from build123d import *

# Parameters (mm, degrees)
SKETCH1_W           = 180
SKETCH1_H           = 110
SKETCH1_R           = 42
SKETCH1_R_2         = 18.1
BOSS_EXTRUDE1_DEPTH = 6
SKETCH3_R           = 1
CUT_EXTRUDE1_DEPTH  = 30


with BuildPart() as part:
    # Sketch1 → Boss-Extrude1 (new body)
    with BuildSketch(Plane.XY):
        with Locations((90, 55)):
            Rectangle(SKETCH1_W, SKETCH1_H)
        with Locations((60, 50)):
            Circle(SKETCH1_R, mode=Mode.SUBTRACT)
        with Locations((140, 60)):
            Circle(SKETCH1_R_2, mode=Mode.SUBTRACT)
    extrude(amount=BOSS_EXTRUDE1_DEPTH)

    # Sketch3 → Cut-Extrude1 (cut)
    with BuildSketch(Plane.XY):
        with Locations((92.880465325, 82.880465325)):
            Circle(SKETCH3_R)
        with Locations((27.119534675, 82.880465325)):
            Circle(SKETCH3_R)
        with Locations((27.119534675, 17.119534675)):
            Circle(SKETCH3_R)
        with Locations((92.880465325, 17.119534675)):
            Circle(SKETCH3_R)
        with Locations((155.202795796, 75.202795796)):
            Circle(SKETCH3_R)
        with Locations((124.797204204, 75.202795796)):
            Circle(SKETCH3_R)
        with Locations((124.797204204, 44.797204204)):
            Circle(SKETCH3_R)
        with Locations((155.202795796, 44.797204204)):
            Circle(SKETCH3_R)
    extrude(amount=CUT_EXTRUDE1_DEPTH, mode=Mode.SUBTRACT)


solid = part.part
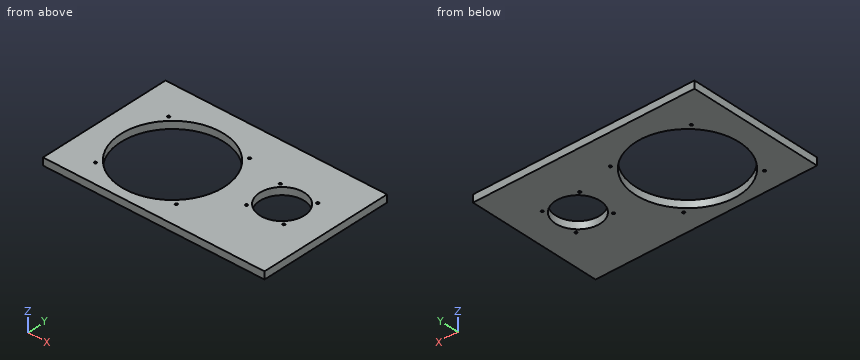
CAD build for the part. Positions are in the model's coordinates, mm. Give positions to 0.01 mm unless a question says otherwise; leave off trailing zeros. Loops run counter-clockwise (first coordinate to the right, second up) from the corner with the lowest first, then second, coordinate; pieces in that order, holes last. Notation, with made-up numbers: M 9,-31.75 L 66,-31.75 A26 cw 66,5.25 Z; hole C 64,48 d4. An arc over 180 degrees is marked long. Write each question's results on one line, items separated by ' | '.
Q1. Band-saw the part on B-B on y = 38. Write the cut outline in (x, z), and give its area (3 significant figures).
Geometry check:
outline: M 0,0 L 19.75,0 L 19.75,6 L 0,6 Z; M 100.25,0 L 180,0 L 180,6 L 100.25,6 Z | area: 597 mm²
Q2. Probe probe 1 along Y at (x, z) = (60, 2.85); probe 2 along Y at (x, z) = (155, 5.45); probe 3 along X at (y, z) = (68.5, 0.7). List the from-to ranges inside material, lowest first.
Geometry check:
probe 1: y = 0 to 8, 92 to 110 | probe 2: y = 0 to 43.82, 45.78 to 49.87, 70.13 to 74.22, 76.18 to 110 | probe 3: x = 0 to 22.29, 97.71 to 124.02, 155.98 to 180
Q3. Band-saw the part on C-C on z = 4.25. Give the number of separate pieces and of enclosed holes in the cut face, and give its area (3 significant figures).
Geometry check:
separate pieces: 1 | enclosed holes: 10 | area: 13,200 mm²
Q4. Band-saw the part on D-D on y = 50. Write the cut outline in (x, z), and give its area (3 significant figures).
Geometry check:
outline: M 0,0 L 18,0 L 18,6 L 0,6 Z; M 102,0 L 124.91,0 L 124.91,6 L 102,6 Z; M 155.09,0 L 180,0 L 180,6 L 155.09,6 Z | area: 395 mm²
Q5. Band-saw the part on A-A on x = 140. Write the cut outline in (y, z).
Geometry check:
outline: M 0,0 L 41.9,0 L 41.9,6 L 0,6 Z; M 78.1,0 L 110,0 L 110,6 L 78.1,6 Z
